from build123d import *

# Parameters (mm, degrees)
BOSS_EXTRUDE1_DEPTH       = 31.75
F_8_CLEARANCE_HOLE1_D     = 4.3053
F_8_CLEARANCE_HOLE1_DEPTH = 6.35
F_8_CLEARANCE_HOLE1_TIP   = 1.293442612
F_8_CLEARANCE_HOLE2_D     = 4.3053
F_8_CLEARANCE_HOLE2_DEPTH = 6.35
F_8_CLEARANCE_HOLE2_TIP   = 1.293442612


with BuildPart() as part:
    # Sketch1 → Boss-Extrude1 (new body)
    with BuildSketch(Plane(origin=(0, 0, 0), x_dir=(1, 0, 0), z_dir=(0, 1, 0))):
        Polygon((0, 0), (120.65, 0), (120.65, -2.794), (2.794, -2.794), (2.794, -120.65), (0, -120.65), align=None)
    extrude(amount=BOSS_EXTRUDE1_DEPTH)

    # #8 Clearance Hole1
    with Locations(Plane(origin=(0, 0, 0), x_dir=(-1, 0, 0), z_dir=(0, 0, -1))):
        with Locations((-107.95, 15.875), (-57.15, 15.875)):
            Hole(F_8_CLEARANCE_HOLE1_D / 2, depth=F_8_CLEARANCE_HOLE1_DEPTH)
            with Locations((0, 0, -(F_8_CLEARANCE_HOLE1_DEPTH + F_8_CLEARANCE_HOLE1_TIP / 2))):  # 118° drill point
                Cone(0, F_8_CLEARANCE_HOLE1_D / 2, F_8_CLEARANCE_HOLE1_TIP, mode=Mode.SUBTRACT)

    # #8 Clearance Hole2
    with Locations(Plane.ZY):
        with Locations((107.95, 15.875), (57.15, 15.875)):
            Hole(F_8_CLEARANCE_HOLE2_D / 2, depth=F_8_CLEARANCE_HOLE2_DEPTH)
            with Locations((0, 0, -(F_8_CLEARANCE_HOLE2_DEPTH + F_8_CLEARANCE_HOLE2_TIP / 2))):  # 118° drill point
                Cone(0, F_8_CLEARANCE_HOLE2_D / 2, F_8_CLEARANCE_HOLE2_TIP, mode=Mode.SUBTRACT)


solid = part.part
For this review, take the finished solid that the model builds, in its own axes (mm). A direction names the side the tool comes from. Give positions to 0.01 mm unless a question says otherwise; leave off trailing zeros. Order: outer loops, then holes, each group sorted by start corner. A loop starts at its lowest first (then second) coordinate and runs counter-clockwise, first axis right, second up. Notation, with made-up numbers: (60.25, -27.5) -> (104.25, -27.5) arc R17 ccw to (104.25, -13.5) -> close; hole circle Ø9 at (41, 6). An arc over 180 degrees is marked (long way). Write item = value, one per line.
1) We need section A-A, the plane z = 57.15. Give the boundary of the cut face in (x, y).
Findings:
outline = (0, 0) -> (2.79, 0) -> (2.79, 13.72) -> (0, 13.72) -> close; (0, 18.03) -> (2.79, 18.03) -> (2.79, 31.75) -> (0, 31.75) -> close
2) We need section C-C, the plane y = 12. Give the boundary of the cut face in (x, z), and give its area (3 significant figures).
Findings:
outline = (0, 0) -> (120.65, 0) -> (120.65, 2.79) -> (2.79, 2.79) -> (2.79, 120.65) -> (0, 120.65) -> close
area = 666 mm^2
3) To check wall thickness, follow L1, parallel to Y at x = 57.15, z = 1.65; L2, parallel to X at y = 8, z = 36.5. State the ranges of each line that lie inside material, in increasing order. Write a range as from..to.
Findings:
L1 = 0..13.72, 18.03..31.75
L2 = 0..2.79
4) Draft analysis for pull direction Z (two halves, no side actions). For faces 3 (the face through (63, 16, 2.794)), 4 (the face through (1.417, 16.522, 55.097)), 5 (the face through (0, 16, 61)), state which applies: pulls with the +Z half, pulls with the -Z half, needs draft (parallel to the pull), parting line crosses it, or undercut.
Findings:
face_3 = pulls with the +Z half
face_4 = undercut
face_5 = needs draft
5) We need section B-B, the plane x = 57.15. Give the boundary of the cut face in (y, z), and give its area (3 significant figures).
Findings:
outline = (0, 0) -> (13.72, 0) -> (13.72, 2.79) -> (0, 2.79) -> close; (18.03, 0) -> (31.75, 0) -> (31.75, 2.79) -> (18.03, 2.79) -> close
area = 76.7 mm^2
6) Insertion check: pin 1 (2 mm diameter, centred on y = 27.5, z = 40.5, fed in from +X); pin 2 (7 mm diameter, centred on x = 57.15, y = 15.875, fed in from +Z); pin 3 (4 mm diameter, centred on x = 107.95, y = 15.875, fed in from +Z). Each pin has a flat end and moves straight along its axis. Give the tip position at first contact, or say it passes through.
Findings:
pin_1 = 2.79
pin_2 = 2.79
pin_3 = through
7) We need section D-D, the plane z = 75. Give the boundary of the cut face in (x, y).
Findings:
outline = (0, 0) -> (2.79, 0) -> (2.79, 31.75) -> (0, 31.75) -> close
8) For faces 1 (the face through (34, 31.75, 2)), 2 (the face through (2.794, 16, 61)), list the 3-axis set-ups (+Z, -Z, +X, -X, +Y, -Y) from which the entire face can be reached by the end or side of a thin tool; tool diameter is ignored.
Findings:
face_1 = +Z, -Z, +X, -X, +Y
face_2 = +Z, +X, +Y, -Y
